Read the model definition and answer for the solid it produces. Units are mm, in the model's axes. A direction names the side the tool comes from. Coordinates: 2 decimals unless noted, no trailing zeros. Loops run counter-clockwise (first coordinate to the right, second up) from the corner with the lowest first, then second, coordinate; pieces in that order, holes last. Notation, with made-up numbers: (12, 70) - (24, 70) arc R26 cw to (24, 101) - close; hole circle Ø3 at (-30.75, 41.5). An arc over 180 degrees is marked (long way). Use one line per item in the form item = value.
from build123d import *

# Parameters (mm, degrees)
SKETCH_1_W             = 30
SKETCH_1_H             = 44.3
EXTRUDE_1_DEPTH        = 6
SKETCH_2_R             = 9
CUT_EXTRUDE_1_DEPTH    = 4.5
SKETCH_3_R             = 7.5
CUT_EXTRUDE_2_DEPTH    = 4.5
SKETCH_5_W             = 8
SKETCH_5_H             = 3.5
CUT_EXTRUDE_3_DEPTH    = 10
FILLET_1_R             = 0.5
SKETCH_6_R             = 1.5
CUT_EXTRUDE_1251_DEPTH = 5


with BuildPart() as part:
    # 草图1 → 凸台-拉伸1 (new body)
    with BuildSketch(Plane(origin=(0, 0, 0), x_dir=(1, 0, 0), z_dir=(0, 1, 0))):
        Rectangle(SKETCH_1_W, SKETCH_1_H)
    extrude(amount=EXTRUDE_1_DEPTH)

    # 草图2 → 切除-拉伸1 (cut)
    with BuildSketch(Plane(origin=(0, 6, 0), x_dir=(1, 0, 0), z_dir=(0, 1, 0))):
        with Locations(Location((0, 11.65, 0), (0, 0, 270))):
            Circle(SKETCH_2_R)
        with Locations(Location((0, -12.15, 0), (0, 0, 270))):
            Circle(SKETCH_2_R)
    extrude(amount=-CUT_EXTRUDE_1_DEPTH, mode=Mode.SUBTRACT)

    # 草图3 → 切除-拉伸2 (cut)
    with BuildSketch(Plane(origin=(0, 1.5, 0), x_dir=(1, 0, 0), z_dir=(0, 1, 0))):
        with Locations(Location((0, 11.65, 0), (0, 0, 270))):
            Circle(SKETCH_3_R)
        with Locations(Location((0, -12.15, 0), (0, 0, 270))):
            Circle(SKETCH_3_R)
    extrude(amount=-CUT_EXTRUDE_2_DEPTH, mode=Mode.SUBTRACT)

    # 草图5 → 切除-拉伸3 (cut)
    with BuildSketch(Plane(origin=(0, 6, 0), x_dir=(1, 0, 0), z_dir=(0, 1, 0))):
        with Locations((11, -20.4)):
            Rectangle(SKETCH_5_W, SKETCH_5_H)
        with Locations((-11, -20.4)):
            Rectangle(SKETCH_5_W, SKETCH_5_H)
    extrude(amount=-CUT_EXTRUDE_3_DEPTH, mode=Mode.SUBTRACT)

    # 圆角1
    fillet_1_edges = [part.edges().sort_by_distance(p)[0] for p in [
        (-7, 3, 18.65),
        (7, 3, 18.65),
    ]]
    fillet(fillet_1_edges, radius=FILLET_1_R)

    # 草图6 → Cut-Extrude 1251 (cut)
    with BuildSketch(Plane.XY.offset(18.65)):
        with Locations((-12, 2)):
            Circle(SKETCH_6_R)
        with Locations(Location((12, 2, 0), (0, 0, 180))):
            Circle(SKETCH_6_R)
    extrude(amount=-CUT_EXTRUDE_1251_DEPTH, mode=Mode.SUBTRACT)


solid = part.part
Item 1: Which of the six approach directions +Z, -Z, +X, -X, +Y, -Y give full straight-line access (tool end or side, diameter ignored) to faces 4 (the flat face through (-12, 2, 13.65)), 5 (the cylindrical face through (2.703, 3.782, -3.066)), 6 (the flat face through (-15, 3, -1)), 7 (the flat face through (-11, 4, 18.65))?
Results below:
face_4 = +Z
face_5 = +Y
face_6 = +Z, -Z, -X, +Y, -Y
face_7 = +Z, -X, +Y, -Y
Item 2: The part is cut by section D-D on x = -12. Give the vertices of the cut face in (y, z).
Results below:
outline = (0, -22.15) - (6, -22.15) - (6, 18.65) - (3.5, 18.65) - (3.5, 13.65) - (0.5, 13.65) - (0.5, 18.65) - (0, 18.65) - close
Item 3: Each of these flat-tipped pins is pushed along its axis until it touches: P1, Ø0.9, axis at x = 12, y = 1.5, coming from the +Z side; P2, Ø3, axis at x = 10, y = 2.5, coming from the +Z side; P3, Ø14.5, axis at x = 0, z = 12.15, coming from the -Y side; P4, Ø1.5, axis at y = 3, z = 21, coming from the -X side. Where does it stop, or does it pass through?
Results below:
P1 = 13.65
P2 = 18.65
P3 = through
P4 = -7
Item 4: For a pull along Y with two mould halves and no side action, classify faces 1 (the flat face through (12, 2, 13.65)), 2 (the flat face through (7, 1.5, -15)), 3 (the flat face through (11, 4, 18.65)) as +Y half, -Y half, draft (parallel to the pull), parting line (faces both ways), or undercut.
Results below:
face_1 = undercut
face_2 = +Y half
face_3 = draft
Item 5: The part is cut by section B-B on x = 0. Give the vertices of the cut face in (y, z), plus the area to 3 significant figures.
Results below:
outline = (0, -22.15) - (6, -22.15) - (6, -20.65) - (1.5, -20.65) - (1.5, -19.15) - (0, -19.15) - close; (0, -4.15) - (1.5, -4.15) - (1.5, -2.65) - (6, -2.65) - (6, 3.15) - (1.5, 3.15) - (1.5, 4.65) - (0, 4.65) - close; (0, 19.65) - (1.5, 19.65) - (1.5, 21.15) - (6, 21.15) - (6, 22.15) - (0, 22.15) - close
area = 58.8 mm²
Item 6: The part is cut by section A-A on z = 12.15. Give the vertices of the cut face in (x, y), plus the area to 3 significant figures.
Results below:
outline = (-15, 0) - (-7.5, 0) - (-7.5, 1.5) - (-9, 1.5) - (-9, 6) - (-15, 6) - close; (7.5, 0) - (15, 0) - (15, 6) - (9, 6) - (9, 1.5) - (7.5, 1.5) - close
area = 76.5 mm²
Item 7: The part is cut by section C-C on y = 5.5. Give the vertices of the cut face in (x, z), plus the area to 3 significant figures.
Results below:
outline = (-15, -22.15) - (15, -22.15) - (15, 18.65) - (7.5, 18.65) arc R0.5 cw to (7, 19.15) - (7, 22.15) - (-7, 22.15) - (-7, 19.15) arc R0.5 cw to (-7.5, 18.65) - (-15, 18.65) - close; hole circle Ø18 at (0, -11.65); hole circle Ø18 at (0, 12.15)
area = 764 mm²
Item 8: Find the intervals of material crossed by L1, parallel to X at y = 1, z = 12.15; L2, parallel to Z at x = -5.5, y = 4.65; L3, parallel to Z at x = -4.75, y = 3.1, in increasing order.
Results below:
L1 = -15 to -7.5, 7.5 to 15
L2 = -22.15 to -18.77, -4.53 to 5.03, 19.27 to 22.15
L3 = -22.15 to -19.29, -4.01 to 4.51, 19.79 to 22.15
